Design review of the part built by this model. Coordinates are the model's own, in mm. Coordinates: 2 decimals unless noted, no trailing zeros. Loops run counter-clockwise (first coordinate to the right, second up) from the corner with the lowest first, then second, coordinate; pieces in that order, holes last. Notation, with made-up numbers: (28, 62.25) - (84, 62.25) arc R15 cw to (84, 68.25) - close; hole circle Ø3 at (39, 80.5). An arc over 180 degrees is marked (long way). Answer in a Markdown table with one row per item. Add a question column.
(1) We need section B-B, the plane z = 0. Write out the cut boundary in (x, y).
(2) We need section D-D, the plane x = -66. Write out the cut boundary in (y, z), plus the area to 3 significant figures.
(3) The part is to be moulded in two halves that separate along X. For faces 1 (the face through (-37.42, 1.52, 0.74)), 2 (the face through (-56.258, 1.479, 22.653)), 3 (the face through (-15.57, 1.48, 35.4)), say which applies: released by +X, released by -X, zero draft, split by the parting line, or undercut.
(4) We need section A-A, the plane x = -22.5. Write out the cut boundary in (y, z), plus the area to 3 significant figures.
(5) To check wall thickness, follow L1, parallel to X at y = 1.2, z = 0; L2, parallel to Z at x = -70, y = 1.6; L3, parallel to X at y = 2.5, z = -3. State the ranges of each line that lie inside material, in increasing order. Write a range as [from, to].
(6) We need section C-C, the plane z = 27.5. Write out the cut boundary in (x, y), plus the area to 3 significant figures.
(7) Clearance check with a flat-ended pin moving along its axis: pin 1 (0.5 mm diameter, centred on x = -71.5, y = 2, fed in from -Z). State where the tip first meets the part, or that it passes through.
from build123d import *

# Parameters (mm, degrees)
SKETCH_1_R          = 1.6
EXTRUDE_1_DEPTH     = 3
SKETCH_2_W          = 38
SKETCH_2_H          = 42
CUT_EXTRUDE_1_DEPTH = 124.527324912
CUT_EXTRUDE_2_DEPTH = 90.235643103
SKETCH_4_W          = 9
SKETCH_4_H          = 18
SKETCH_4_W_2        = 15
SKETCH_4_H_2        = 9
CUT_EXTRUDE_3_DEPTH = 90.235643103
SKETCH_5_W          = 44
SKETCH_5_H          = 4
EXTRUDE_2_DEPTH     = 3
SKETCH_6_W          = 4
SKETCH_6_H          = 15.328304062
EXTRUDE_3_DEPTH     = 3
SKETCH_7_R          = 2
CUT_EXTRUDE_4_DEPTH = 86.0529247
EXTRUDE_4_DEPTH     = 3
FILLET_2_R          = 2
FILLET_1_R          = 1.5
SKETCH_9_R          = 1.6
CUT_EXTRUDE_5_DEPTH = 86.0529247
SKETCH_10_R         = 4
SKETCH_10_R_2       = 1.6
EXTRUDE_5_DEPTH     = 3
FILLET_3_R          = 1.5


with BuildPart() as part:
    # 草图1 → 凸台-拉伸1 (new body)
    with BuildSketch(Plane(origin=(0, 0, 0), x_dir=(1, 0, 0), z_dir=(0, 1, 0))):
        Polygon((-30, 39.804513537), (-30, 45), (-15, 45), (-15, -45), (-30, -45), (-30, -39.804513537), (-30, -21), (-96.599318778, -21), (-115, -21), (-115, 21), (-96.599318778, 21), (-30, 21), align=None)
        with Locations(Location((-71, -17, 0), (0, 0, 270))):
            Circle(SKETCH_1_R, mode=Mode.SUBTRACT)
        with Locations(Location((-71, 17, 0), (0, 0, 270))):
            Circle(SKETCH_1_R, mode=Mode.SUBTRACT)
        with Locations(Location((-22.5, 30, 0), (0, 0, 270))):
            Circle(SKETCH_1_R, mode=Mode.SUBTRACT)
        with Locations(Location((-22.5, -30, 0), (0, 0, 270))):
            Circle(SKETCH_1_R, mode=Mode.SUBTRACT)
        with Locations(Location((-22.5, 0, 0), (0, 0, 270))):
            Circle(SKETCH_1_R, mode=Mode.SUBTRACT)
    extrude(amount=EXTRUDE_1_DEPTH)

    # 草图2 → 切除-拉伸1 (cut, through all)
    with BuildSketch(Plane(origin=(0, 3, 0), x_dir=(1, 0, 0), z_dir=(0, 1, 0))):
        with Locations((-96, 0)):
            Rectangle(SKETCH_2_W, SKETCH_2_H)
    extrude(amount=-CUT_EXTRUDE_1_DEPTH, mode=Mode.SUBTRACT)

    # 草图3 → 切除-拉伸2 (cut, through all)
    with BuildSketch(Plane(origin=(0, 3, 0), x_dir=(1, 0, 0), z_dir=(0, 1, 0))):
        Polygon((-68.016430897, 13), (-74, 13), (-74, -13), (-68.016430897, -13), (-65, -10.328304062), (-65, 10.328304062), align=None)
        Polygon((-53.339011543, 0), (-65, 10.328304062), (-65, -10.328304062), align=None)
        Polygon((-65, 18), (-65, 15.671695938), (-50.322580645, 2.671695938), (-33.016430897, 18), align=None)
        Polygon((-30, 15.328304062), (-47.306149748, 0), (-30, -15.328304062), align=None)
        Polygon((-50.322580645, -2.671695938), (-65, -15.671695938), (-65, -18), (-33.016430897, -18), align=None)
    extrude(amount=-CUT_EXTRUDE_2_DEPTH, mode=Mode.SUBTRACT)

    # 草图4 → 切除-拉伸3 (cut, through all)
    with BuildSketch(Plane(origin=(0, 3, 0), x_dir=(1, 0, 0), z_dir=(0, 1, 0))):
        with Locations((-22.5, 15)):
            Rectangle(SKETCH_4_W, SKETCH_4_H)
        with Locations((-22.5, 40.5)):
            Rectangle(SKETCH_4_W_2, SKETCH_4_H_2)
        with Locations((-22.5, -40.5)):
            Rectangle(SKETCH_4_W_2, SKETCH_4_H_2)
        with Locations((-22.5, -15)):
            Rectangle(SKETCH_4_W, SKETCH_4_H)
    extrude(amount=-CUT_EXTRUDE_3_DEPTH, mode=Mode.SUBTRACT)

    # 草图5 → 凸台-拉伸2 (add)
    with BuildSketch(Plane(origin=(0, 3, 0), x_dir=(1, 0, 0), z_dir=(0, 1, 0))):
        with Locations((-52, 0)):
            Rectangle(SKETCH_5_W, SKETCH_5_H)
    extrude(amount=-EXTRUDE_2_DEPTH)

    # 草图6 → 凸台-拉伸3 (add)
    with BuildSketch(Plane(origin=(0, 3, 0), x_dir=(1, 0, 0), z_dir=(0, 1, 0))):
        with Locations((-50.322580645, -10.335847969)):
            Rectangle(SKETCH_6_W, SKETCH_6_H)
        with Locations((-50.322580645, 10.335847969)):
            Rectangle(SKETCH_6_W, SKETCH_6_H)
    extrude(amount=-EXTRUDE_3_DEPTH)

    # 草图7 → 切除-拉伸4 (cut, through all)
    with BuildSketch(Plane(origin=(0, 3, 0), x_dir=(1, 0, 0), z_dir=(0, 1, 0))):
        with Locations(Location((-50.322580645, 0, 0), (0, 0, 270))):
            Circle(SKETCH_7_R)
    extrude(amount=-CUT_EXTRUDE_4_DEPTH, mode=Mode.SUBTRACT)

    # 草图8 → 凸台-拉伸4 (add)
    with BuildSketch(Plane(origin=(0, 3, 0), x_dir=(1, 0, 0), z_dir=(0, 1, 0))):
        Polygon((-77, 21), (-30, 36), (-30, 32.850920072), (-67.132882893, 21), align=None)
        Polygon((-67.132882893, -21), (-77, -21), (-30, -36), (-30, -32.850920072), align=None)
    extrude(amount=-EXTRUDE_4_DEPTH)

    # 圆角2
    fillet_2_edges = [part.edges().sort_by_distance(p)[0] for p in [
        (-74, 1.5, -13),
        (-68.016430897, 1.5, -13),
        (-30, 1.5, -36),
        (-15, 1.5, -36),
        (-30, 1.5, 36),
        (-15, 1.5, 36),
        (-18, 1.5, 24),
        (-27, 1.5, 24),
        (-27, 1.5, 6),
        (-18, 1.5, 6),
        (-27, 1.5, -6),
        (-27, 1.5, -24),
        (-18, 1.5, -24),
        (-18, 1.5, -6),
        (-55.597076059, 1.5, -2),
        (-74, 1.5, -2),
        (-55.597076059, 1.5, 2),
        (-74, 1.5, 2),
        (-48.322580645, 1.5, -4.443124509),
        (-48.322580645, 1.5, 4.443124509),
        (-48.322580645, 1.5, 18),
        (-52.322580645, 1.5, 4.443124509),
        (-52.322580645, 1.5, 18),
        (-30, 1.5, 21),
        (-30, 1.5, -21),
        (-48.322580645, 1.5, -18),
        (-52.322580645, 1.5, -4.443124509),
        (-52.322580645, 1.5, -18),
        (-67.132882893, 1.5, -21),
        (-30, 1.5, -32.850920072),
        (-67.132882893, 1.5, 21),
        (-30, 1.5, 32.850920072),
        (-77, 1.5, -21),
        (-77, 1.5, 21),
        (-30, 1.5, -15.328304062),
        (-30, 1.5, 15.328304062),
        (-33.016430897, 1.5, -18),
        (-33.016430897, 1.5, 18),
        (-68.016430897, 1.5, 13),
        (-74, 1.5, 13),
    ]]
    fillet(fillet_2_edges, radius=FILLET_2_R)

    # 圆角1
    fillet_1_edges = [part.edges().sort_by_distance(p)[0] for p in [
        (-65, 1.5, -15.671695938),
        (-65, 1.5, -18),
        (-65, 1.5, 15.671695938),
        (-65, 1.5, 18),
    ]]
    fillet(fillet_1_edges, radius=FILLET_1_R)

    # 草图9 → 切除-拉伸5 (cut, through all)
    with BuildSketch(Plane(origin=(0, 3, 0), x_dir=(1, 0, 0), z_dir=(0, 1, 0))):
        with Locations(Location((-36, 0, 0), (0, 0, 270))):
            Circle(SKETCH_9_R)
        with Locations(Location((-66, 0, 0), (0, 0, 270))):
            Circle(SKETCH_9_R)
    extrude(amount=-CUT_EXTRUDE_5_DEPTH, mode=Mode.SUBTRACT)

    # 草图10 → 凸台-拉伸5 (add)
    # profile 1 of 2: a face of its own
    with BuildSketch(Plane(origin=(0, 3, 0), x_dir=(1, 0, 0), z_dir=(0, 1, 0))):
        with Locations((-66, 0)):
            Circle(SKETCH_10_R)
        with Locations(Location((-66, 0, 0), (0, 0, 270))):
            Circle(SKETCH_10_R_2, mode=Mode.SUBTRACT)
    # profile 2 of 2: a face of its own
    with BuildSketch(Plane(origin=(0, 3, 0), x_dir=(1, 0, 0), z_dir=(0, 1, 0))):
        with Locations((-36, 0)):
            Circle(SKETCH_10_R)
        with Locations(Location((-36, 0, 0), (0, 0, 270))):
            Circle(SKETCH_10_R_2, mode=Mode.SUBTRACT)
    extrude(amount=-EXTRUDE_5_DEPTH)

    # 圆角3
    fillet_3_edges = [part.edges().sort_by_distance(p)[0] for p in [
        (-45.048085232, 1.5, 2),
        (-30, 1.5, 2),
        (-30, 1.5, -2),
        (-45.048085232, 1.5, -2),
        (-69.464101615, 1.5, 2),
        (-62.535898385, 1.5, 2),
        (-32.535898385, 1.5, -2),
        (-39.464101615, 1.5, -2),
        (-69.464101615, 1.5, -2),
        (-62.535898385, 1.5, -2),
        (-32.535898385, 1.5, 2),
        (-39.464101615, 1.5, 2),
    ]]
    fillet(fillet_3_edges, radius=FILLET_3_R)


solid = part.part
Responses:
| question | item | result |
|---|---|---|
| 1 | outline | (-77, 0) - (-67.6, 0) - (-67.6, 3) - (-77, 3) - close; (-64.4, 0) - (-52.32, 0) - (-52.32, 3) - (-64.4, 3) - close; (-48.32, 0) - (-37.6, 0) - (-37.6, 3) - (-48.32, 3) - close; (-34.4, 0) - (-24.1, 0) - (-24.1, 3) - (-34.4, 3) - close; (-20.9, 0) - (-15, 0) - (-15, 3) - (-20.9, 3) - close |
| 2 | outline | (0, -24.51) - (3, -24.51) - (3, -11.21) - (0, -11.21) - close; (0, -4) - (3, -4) - (3, -1.6) - (0, -1.6) - close; (0, 1.6) - (3, 1.6) - (3, 4) - (0, 4) - close; (0, 11.21) - (3, 11.21) - (3, 24.51) - (0, 24.51) - close |
| 2 | area | 94.2 mm2 |
| 3 | face 1 | undercut |
| 3 | face 2 | undercut |
| 3 | face 3 | released by +X |
| 4 | outline | (0, -36) - (3, -36) - (3, -31.6) - (0, -31.6) - close; (0, -28.4) - (3, -28.4) - (3, -24) - (0, -24) - close; (0, -6) - (3, -6) - (3, -1.6) - (0, -1.6) - close; (0, 1.6) - (3, 1.6) - (3, 6) - (0, 6) - close; (0, 24) - (3, 24) - (3, 28.4) - (0, 28.4) - close; (0, 31.6) - (3, 31.6) - (3, 36) - (0, 36) - close |
| 4 | area | 79.2 mm2 |
| 5 | L1 | x = [-77, -67.6], [-64.4, -52.32], [-48.32, -37.6], [-34.4, -24.1], [-20.9, -15] |
| 5 | L2 | z = [-23.23, -18.25], [-15.75, -13], [-2.02, 2.02], [13, 15.75], [18.25, 23.23] |
| 5 | L3 | x = [-77, -73.73], [-68.65, -63.35], [-59.14, -42.51], [-38.65, -33.35], [-30.09, -15] |
| 6 | outline | (-56.63, 0) - (-46.77, 0) - (-46.77, 3) - (-56.63, 3) - close; (-30, 0) - (-15, 0) - (-15, 3) - (-30, 3) - close |
| 6 | area | 74.6 mm2 |
| 7 | pin 1 | stops at z = -22.84 |
